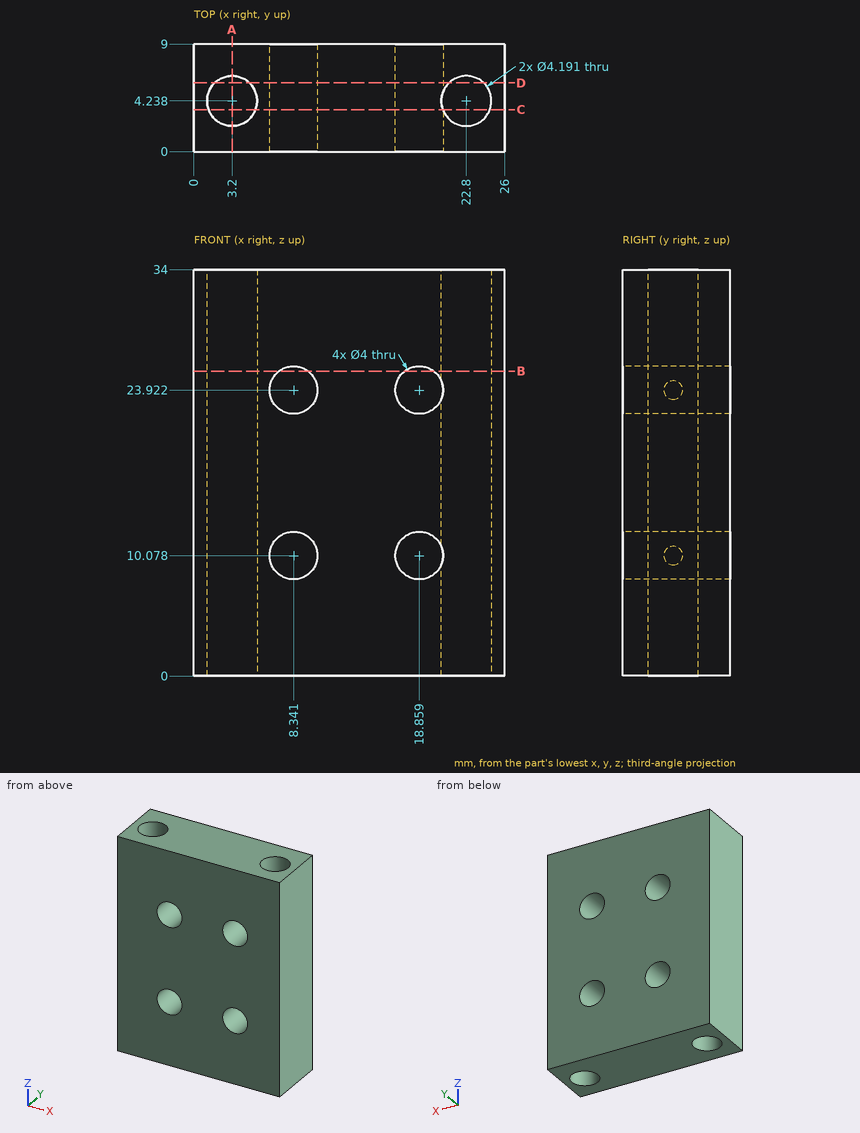
Design review of the part shown in the three views and the two pictorial views. Dimensions are in mm from the part's minimum x, y and z. Give positions to 0.01 mm unless a question says otherwise; leave off trailing zeros. Write each loop counter-clockwise with the first axis right and the second up, starting at its lowest first coordinate (ties: lowest second). Pieces come first, ordered by that corner, then holes. Notation, with made-up numbers: (43, 29) -> (79, 29) arc R30 ccw to (79, 61) -> close; hole circle Ø1 at (2.25, 88.25). An arc over 180 degrees is marked (long way). Answer in a Markdown table with one row per item.
1) Add section D-D on y = 5.75. State the section outline as (x, z) points.
Worked answers:
| item | result |
|---|---|
| outline | (0, 0) -> (1.75, 0) -> (1.75, 34) -> (0, 34) -> close; (4.65, 0) -> (21.35, 0) -> (21.35, 34) -> (4.65, 34) -> close; (24.25, 0) -> (26, 0) -> (26, 34) -> (24.25, 34) -> close; hole circle Ø4 at (8.34, 10.08); hole circle Ø4 at (8.34, 23.92); hole circle Ø4 at (18.86, 10.08); hole circle Ø4 at (18.86, 23.92) |
2) Add section C-C on y = 3.5. State the section outline as (x, z) points.
Worked answers:
| item | result |
|---|---|
| outline | (0, 0) -> (1.24, 0) -> (1.24, 34) -> (0, 34) -> close; (5.16, 0) -> (20.84, 0) -> (20.84, 9.79) arc R2 cw (long way) to (20.84, 10.36) -> (20.84, 23.64) arc R2 cw (long way) to (20.84, 24.21) -> (20.84, 34) -> (5.16, 34) -> close; (24.76, 0) -> (26, 0) -> (26, 34) -> (24.76, 34) -> close; hole circle Ø4 at (8.34, 10.08); hole circle Ø4 at (8.34, 23.92) |
3) Add section A-A on x = 3.2. State the section outline as (y, z) points.
Worked answers:
| item | result |
|---|---|
| outline | (0, 0) -> (2.14, 0) -> (2.14, 34) -> (0, 34) -> close; (6.33, 0) -> (9, 0) -> (9, 34) -> (6.33, 34) -> close |
4) Clearance check with a flat-ended pin moving along its axis: P1, Ø4.5, axis at x = 8.34, z = 10.08, coming from the -Y side. State where the tip first meets the part, or that it passes through.
Worked answers:
| item | result |
|---|---|
| P1 | y = 0 |
5) For L1, parallel to X at y = 1, z = 23 (1 decimal); L2, parallel to X at y = 6.5, z = 24; L3, parallel to Y at x = 22.8, z = 19, list the stretches that pass through material, from the lowest coordinate up. Write a range as [from, to].
Worked answers:
| item | result |
|---|---|
| L1 | [0, 6.6], [10.1, 17.1], [20.6, 26] |
| L2 | [0, 6.34], [10.34, 16.86], [20.86, 26] |
| L3 | [0, 2.14], [6.33, 9] |
6) Add section B-B on z = 25.5. State the section outline as (x, y) points (1 decimal), plus the area to 3 significant figures.
Worked answers:
| item | result |
|---|---|
| outline | (0, 0) -> (7.1, 0) -> (7.1, 9) -> (0, 9) -> close; (9.6, 0) -> (17.6, 0) -> (17.6, 9) -> (9.6, 9) -> close; (20.1, 0) -> (26, 0) -> (26, 9) -> (20.1, 9) -> close; hole circle Ø4.2 at (3.2, 4.2); hole circle Ø4.2 at (22.8, 4.2) |
| area | 162 mm² |
